from build123d import *

# Parameters (mm, degrees)
POCKET005_DEPTH         = 0.3
POLARPATTERN001_COUNT   = 2
POLARPATTERN001_ANGLE   = 90
BODY015_PLACEMENT_ANGLE = 180


with BuildPart() as part:
    # Sketch028 → Revolution001 (revolve)
    with BuildSketch(Plane.XZ):
        Polygon((0, 0), (0, -10), (1.5, -1.25), (2.65, -0.1), (2.65, 0), align=None)
    revolve(axis=Axis((0, 0, 0), (0, 0, 1)))

    # Sketch029 → Pocket005 (cut, symmetric)
    with BuildSketch(Plane.XZ):
        Polygon((-2, 0), (0, -2), (2, 0), align=None)
    pocket005 = extrude(amount=POCKET005_DEPTH, both=True, mode=Mode.SUBTRACT)

    # PolarPattern001: Pocket005 ×2 about axis
    polarpattern001_axis = Axis((0, 0, 0), (0, 0, 1))
    for i in range(1, POLARPATTERN001_COUNT):
        add(pocket005.rotate(polarpattern001_axis, i * POLARPATTERN001_ANGLE / (POLARPATTERN001_COUNT - 1)), mode=Mode.SUBTRACT)


with BuildPart() as part_1:
    # Body015 placement: moved
    add(part.part.moved(Location((-30, 55, -6))).rotate(Axis((-30, 55, -6), (0, 1, 0)), BODY015_PLACEMENT_ANGLE))


solid = part_1.part
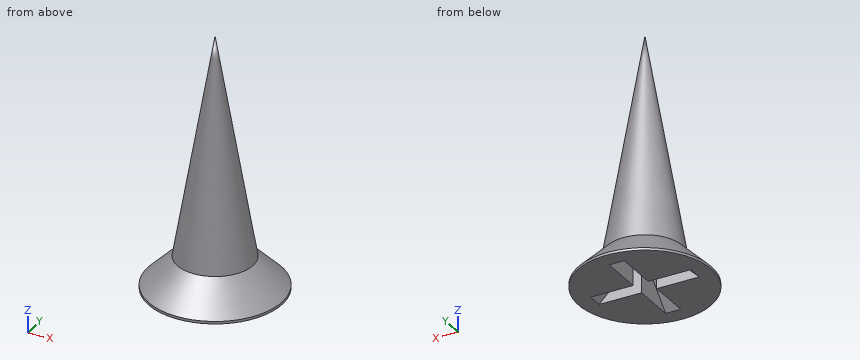
Design review of the part built by this model. Coordinates are the model's own, in mm. Round coordinates to 2 decimals unless told otherwise and drop trailing zeros. Loops run counter-clockwise (first coordinate to the right, second up) from the corner with the lowest first, then second, coordinate; pieces in that order, holes last. Notation, with made-up numbers: (46.25, -33.5) - (99.25, -33.5) arc R21 ccw to (99.25, -29.5) - close; hole circle Ø11 at (77.5, 32.25). An arc over 180 degrees is marked (long way). One line per question, with ' | ' between items.
1. We need section A-A, the plane z = 2.25. State the section outline as (x, y) points, and give its area (3 significant figures).
Results are:
outline: circle Ø0.6 at (-30, 55) | area: 0.283 mm²
2. Clearance check with flat-ended pins moving along their axes: P1, Ø0.5, axis at x = -31.5, z = -5.5, coming from the -Y side; P2, Ø0.8, axis at y = 54, z = -5, coming from the +X side; P3, Ø1.9, axis at y = 56.5, z = -5.5, coming from the -X side; P4, Ø1.5, axis at x = -31.5, z = 1.5, coming from the +Y side. State where each tip first meets the part, or that it passes through.
Results are:
P1: stops at y = 52.95 | P2: stops at x = -28.06 | P3: stops at x = -32.57 | P4: passes through
3. For L1, parallel to Z at x = -31.9, y = 53.65; L2, parallel to Z at x = -28.7, y = 53.15; L3, parallel to Y at x = -30.4, z = 1, list the stretches that pass through material, from the lowest coordinate up. Write a range as [from, to].
Results are:
L1: z = [-6, -5.58] | L2: z = [-6, -5.51] | L3: y = [54.68, 55.32]
4. We need section B-B, the plane z = -2.5. State the section outline as (x, y) points, and give its area (3 significant figures).
Results are:
outline: circle Ø2.23 at (-30, 55) | area: 3.90 mm²
